from build123d import *

# Parameters (mm, degrees)
F4_DEPTH = 127
F3_W     = 50.8
F3_H     = 50.8
F5_DEPTH = 127


with BuildPart() as f1:
    # F0 (on Front) → F1 (revolve)
    with BuildSketch(Plane.XZ):
        with BuildLine():
            Line((0, 0), (0, -76.2))
            ThreePointArc((0, -76.2), (76.2, 0), (0, 76.2))
            Line((0, 76.2), (0, 0))
        make_face()
    revolve(axis=Axis((0, 0, 0), (0, 0, -1)))

    # F2 (on Front) → F4 (cut, symmetric)
    with BuildSketch(Plane.XZ):
        with BuildLine():
            Line((-25.4, 25.4), (-25.4, 71.8420489686))
            ThreePointArc((-25.4, 71.8420489686), (-53.8815367264, 53.8815367264), (-71.8420489686, 25.4))
            Line((-71.8420489686, 25.4), (-25.4, 25.4))
        make_face()
        with BuildLine():
            Line((-25.4, -25.4), (-25.4, 25.4))
            Line((-25.4, 25.4), (-71.8420489686, 25.4))
            ThreePointArc((-71.8420489686, 25.4), (-76.2, 0), (-71.8420489686, -25.4))
            Line((-71.8420489686, -25.4), (-25.4, -25.4))
        make_face()
        with BuildLine():
            ThreePointArc((-71.8420489686, -25.4), (-53.8815367264, -53.8815367264), (-25.4, -71.8420489686))
            Line((-25.4, -71.8420489686), (-25.4, -25.4))
            Line((-25.4, -25.4), (-71.8420489686, -25.4))
        make_face()
        with BuildLine():
            ThreePointArc((-25.4, -71.8420489686), (0, -76.2), (25.4, -71.8420489686))
            Line((25.4, -71.8420489686), (25.4, -25.4))
            Line((25.4, -25.4), (-25.4, -25.4))
            Line((-25.4, -25.4), (-25.4, -71.8420489686))
        make_face()
        with BuildLine():
            ThreePointArc((25.4, -71.8420489686), (53.8815367264, -53.8815367264), (71.8420489686, -25.4))
            Line((71.8420489686, -25.4), (25.4, -25.4))
            Line((25.4, -25.4), (25.4, -71.8420489686))
        make_face()
        with BuildLine():
            ThreePointArc((71.8420489686, -25.4), (75.1026102456, -12.8855707789), (76.2, 0))
            ThreePointArc((76.2, 0), (75.1026102456, 12.8855707789), (71.8420489686, 25.4))
            Line((71.8420489686, 25.4), (25.4, 25.4))
            Line((25.4, 25.4), (25.4, -25.4))
            Line((25.4, -25.4), (71.8420489686, -25.4))
        make_face()
        with BuildLine():
            Line((25.4, 25.4), (71.8420489686, 25.4))
            ThreePointArc((71.8420489686, 25.4), (53.8815367264, 53.8815367264), (25.4, 71.8420489686))
            Line((25.4, 71.8420489686), (25.4, 25.4))
        make_face()
    extrude(amount=F4_DEPTH, both=True, mode=Mode.SUBTRACT)

    # F3 (on Right) → F5 (cut, symmetric)
    with BuildSketch(Plane.YZ):
        with BuildLine():
            ThreePointArc((71.8420489686, -25.4), (75.1026102456, -12.8855707789), (76.2, 0))
            ThreePointArc((76.2, 0), (75.1026102456, 12.8855707789), (71.8420489686, 25.4))
            Line((71.8420489686, 25.4), (25.4, 25.4))
            Line((25.4, 25.4), (25.4, -25.4))
            Line((25.4, -25.4), (71.8420489686, -25.4))
        make_face()
        with BuildLine():
            Line((25.4, 25.4), (71.8420489686, 25.4))
            ThreePointArc((71.8420489686, 25.4), (53.8815367264, 53.8815367264), (25.4, 71.8420489686))
            Line((25.4, 71.8420489686), (25.4, 25.4))
        make_face()
        Rectangle(F3_W, F3_H)
        with BuildLine():
            ThreePointArc((-25.4, -71.8420489686), (0, -76.2), (25.4, -71.8420489686))
            Line((25.4, -71.8420489686), (25.4, -25.4))
            Line((25.4, -25.4), (-25.4, -25.4))
            Line((-25.4, -25.4), (-25.4, -71.8420489686))
        make_face()
        with BuildLine():
            Line((-25.4, 25.4), (-25.4, 71.8420489686))
            ThreePointArc((-25.4, 71.8420489686), (-53.8815367264, 53.8815367264), (-71.8420489686, 25.4))
            Line((-71.8420489686, 25.4), (-25.4, 25.4))
        make_face()
        with BuildLine():
            Line((-25.4, -25.4), (-25.4, 25.4))
            Line((-25.4, 25.4), (-71.8420489686, 25.4))
            ThreePointArc((-71.8420489686, 25.4), (-76.2, 0), (-71.8420489686, -25.4))
            Line((-71.8420489686, -25.4), (-25.4, -25.4))
        make_face()
    extrude(amount=F5_DEPTH, both=True, mode=Mode.SUBTRACT)

    # F6 (on Front) → F7 (revolve, cut)
    with BuildSketch(Plane.XZ):
        with BuildLine():
            Line((0, 0), (50.8, 0))
            ThreePointArc((50.8, 0), (0, 50.8), (-50.8, 0))
            Line((-50.8, 0), (0, 0))
        make_face()
    revolve(axis=Axis((25.4, 0, 0), (1, 0, 0)), mode=Mode.SUBTRACT)


solid = f1.part
The listing builds one solid part. Answer for the finished solid, in the listing's coordinates (mm). Give positions to 0.01 mm unless a question says otherwise; leave off trailing zeros. Loops run counter-clockwise (first coordinate to the right, second up) from the corner with the lowest first, then second, coordinate; pieces in that order, holes last.
Item 1: Find the intervals of material crossed by line 1 along X through (y, z) = (-3, 46.5); line 2 along X through (y, z) = (15.5, 42.5); line 3 along Z through (x, y) = (14.5, 4.5), in increasing order.
Derived:
line 1: x = -25.4 to -20.23, 20.23 to 25.4
line 2: x = -25.4 to -23.11, 23.11 to 25.4
line 3: z = 48.48 to 74.67
Item 2: This flat-tipped pin is pushed along its axis until it touches: pin 1 Ø12 at (x, y) = (-0.5, 15.5) entering from +Z. Where does it stop, or does it pass through?
Derived:
pin 1: stops at z = 75.6
Item 3: A cutting plane is placed at C-C (x = 18.5). Give the vertices of the cut face in (y, z), then the cut area to 3 significant figures.
Derived:
outline: (-25.4, 39.92) arc R47.31 cw to (25.4, 39.92) - (25.4, 69.42) arc R73.92 ccw to (-25.4, 69.42) - close
area: 1,400 mm2
Item 4: A cutting plane is placed at D-D (y = -8.5). Give the vertices of the cut face in (x, z).
Derived:
outline: (-25.4, 43.17) arc R50.08 cw to (25.4, 43.17) - (25.4, 71.34) arc R75.72 ccw to (-25.4, 71.34) - close
Item 5: A cutting plane is placed at A-A (z = 41). Give the vertices of the cut face in (x, y).
Derived:
outline: (-25.4, -25.4) - (-15.95, -25.4) arc R29.99 cw to (-25.4, -15.95) - close; (-25.4, 15.95) arc R29.99 cw to (-15.95, 25.4) - (-25.4, 25.4) - close; (15.95, -25.4) - (25.4, -25.4) - (25.4, -15.95) arc R29.99 cw to start; (15.95, 25.4) arc R29.99 cw to (25.4, 15.95) - (25.4, 25.4) - close
Item 6: A cutting plane is placed at B-B (z = 46). Give the vertices of the cut face in (x, y), then the cut area to 3 significant figures.
Derived:
outline: (-25.4, -25.4) - (25.4, -25.4) - (25.4, 25.4) - (-25.4, 25.4) - close; hole circle Ø43.11 at (0, 0)
area: 1,120 mm2
